Answer from the drawing. Dimensions are ordinates in mm from the lowest x, y and z of the part. Give positions to 0.01 mm unless a question says otherwise; leave off trailing zeros. Write each loop counter-clockwise with the first axis right and the second up, starting at its lowest first coordinate (ties: lowest second). Pieces come first, ordered by that corner, then holes.
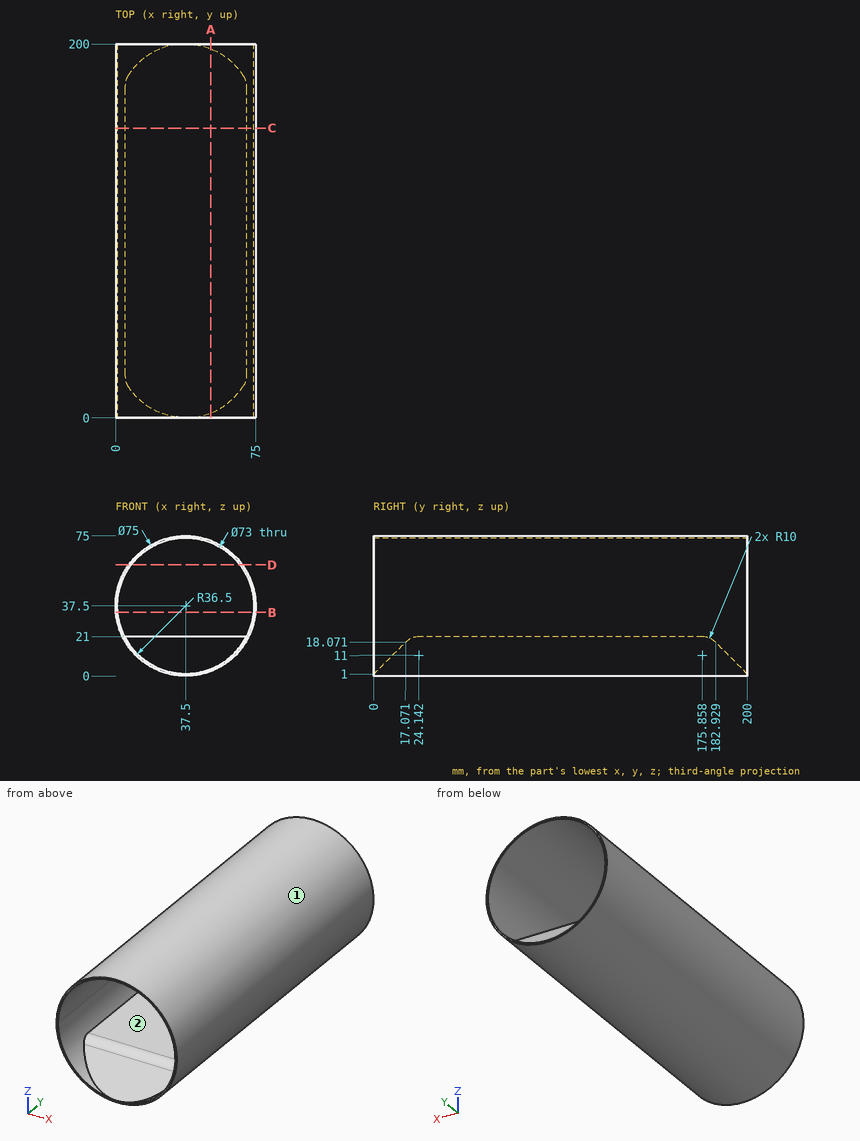
Item 1: Section B-B (z = 34) is taken. Write down the section's boundary in (x, y), and give its area (3 significant figures).
Result set:
outline: (0.16, 0) - (1.17, 0) - (1.17, 200) - (0.16, 200) - close; (73.83, 0) - (74.84, 0) - (74.84, 200) - (73.83, 200) - close
area: 402 mm2
Item 2: Find the intervals of material crossed by line 1 along X through (y, z) = (110.5, 37.5); line 2 along Z through (x, y) = (37, 142); line 3 along Z through (x, y) = (14, 12), in increasing order.
Result set:
line 1: x = 0 to 1, 74 to 75
line 2: z = 0 to 21, 74 to 75
line 3: z = 8.28 to 13, 65.43 to 66.72
Item 3: Section C-C (y = 155) is taken. Write down the section's boundary in (x, z).
Result set:
outline: circle Ø75 at (37.5, 37.5); hole (4.94, 21) - (70.06, 21) arc R36.5 ccw (long way) to start
Item 4: Each of these flat-tipped pins is pushed along its axis until it touches: pin 1 Ø10 at (x, z) = (21, 16) entering from -Y; pin 2 Ø3 at (x, y) = (31.5, 67.5) entering from +Z; pin 3 Ø5 at (y, z) = (36, 63.5) entering from -X. Where does it stop, or does it pass through?
Result set:
pin 1: stops at y = 10
pin 2: stops at z = 74.73
pin 3: stops at x = 8.28
Item 5: Section A-A (x = 51) is taken. Write down the section's boundary in (y, z).
Result set:
outline: (0, 2.51) - (200, 2.51) - (200, 3.59) - (197.41, 3.59) - (182.93, 18.07) arc R10 ccw to (175.86, 21) - (24.14, 21) arc R10 ccw to (17.07, 18.07) - (2.59, 3.59) - (0, 3.59) - close; (0, 71.41) - (200, 71.41) - (200, 72.49) - (0, 72.49) - close
Item 6: Determine the mould class of the marked faces 1 and 2 for opening direction Z: pulls with the +Z half, pulls with the -Z half, needs draft (parallel to the pull), parting line crosses it, or undercut.
Result set:
face 1: parting line crosses it
face 2: undercut
Item 7: Section D-D (z = 59.5) is taken. Write down the section's boundary in (x, y) (1 decimal).
Result set:
outline: (7.1, 0) - (8.4, 0) - (8.4, 200) - (7.1, 200) - close; (66.6, 0) - (67.9, 0) - (67.9, 200) - (66.6, 200) - close
